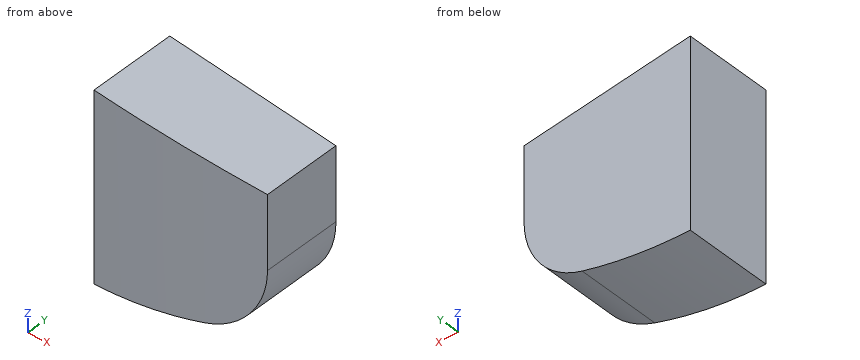
from build123d import *

# Parameters (mm, degrees)
F5_DEPTH = 65
F6_DEPTH = 100


with BuildPart() as f5:
    # F0 (on Front) → F5 (new body)
    with BuildSketch(Plane.XZ):
        with BuildLine():
            Line((0, 22.5), (-102, 32.5))
            Line((-102, 32.5), (-102, -82.5))
            ThreePointArc((-102, -82.5), (-68.454124, -78.918769), (-35.66207, -70.992093))
            ThreePointArc((-35.66207, -70.992093), (-9.875393, -52.596787), (0, -22.5))
            Line((0, -22.5), (0, 22.5))
        make_face()
    extrude(amount=F5_DEPTH)

    # F4 (on Top) → F6 (intersect, symmetric)
    with BuildSketch(Plane.XY):
        with BuildLine():
            Line((0, 0), (-102, 0))
            Line((-102, 0), (-102, -52.5))
            ThreePointArc((-102, -52.5), (-50.938762, -51.24925), (0, -47.5))
            Line((0, -47.5), (0, -22.5))
            Line((0, -22.5), (0, 0))
        make_face()
    extrude(amount=F6_DEPTH, both=True, mode=Mode.INTERSECT)


solid = f5.part
The listing builds one solid part. Answer for the finished solid, in the listing's coordinates (mm). Round coordinates to 2 decimals unless told otherwise and drop trailing zeros. Write each loop counter-clockwise with the first axis right and the second up, starting at its lowest first coordinate (ties: lowest second). Pieces come first, ordered by that corner, then holes. Notation, with made-up numbers: M 55.5,-27.75 L 90.5,-27.75 A21 ccw 90.5,-11.75 Z; hole C -9.75,47 d9. An arc over 180 degrees is marked long. Write each question's results on one line, items separated by ' | '. Start each with the question number.
(1) The part is cut by section A-A, the plane y = -8.5. Write down the section's boundary in (x, z).
(2) Find the intervals of material crossed by line 1 (Y direction, x = -44, z = -27.5); line 2 (Y direction, x = -31, z = -30.5); line 3 (Z direction, x = -41, y = -28.5), in increasing order.
(3) The part is cut by section B-B, the plane z = -21. Write down the section's boundary in (x, y).
(4) The part is cut by section C-C, the plane x = -78. Write down the section's boundary in (y, z).
(5) Each of these flat-tipped pins is pushed along its axis until it touches: P1, Ø6, axis at x = -27.5, y = -21.5, coming from the +Z side; P2, Ø5, axis at x = -31.5, z = -40, coming from the +Y side; P3, Ø12, axis at x = -51.5, y = -35, coming from the -Z side; P4, Ø4, axis at x = -26, z = -34, coming from the -Y side. Where does it stop, or does it pass through?
Worked answers:
1) outline: M -102,-82.5 A258.06 ccw -35.66,-70.99 A50.8 ccw 0,-22.5 L 0,22.5 L -102,32.5 Z
2) line 1: y = -50.89 to 0 | line 2: y = -50.08 to 0 | line 3: z = -72.6 to 26.52
3) outline: M -102,-52.5 A1042.9 ccw 0,-47.5 L 0,0 L -102,0 Z
4) outline: M -52.22,-80.39 L 0,-80.39 L 0,30.15 L -52.22,30.15 Z
5) P1: stops at z = 25.49 | P2: stops at y = 0 | P3: stops at z = -76.77 | P4: stops at y = -49.87
